Verification items for the finished model (mm, model axes). A direction names the side the tool comes from. Round coordinates to 2 decimals unless told otherwise and drop trailing zeros. Write each loop counter-clockwise with the first axis right and the second up, starting at its lowest first coordinate (ties: lowest second). Pieces come first, ordered by that corner, then holes. Notation, with made-up numbers: (31.25, 19) -> (78.25, 19) arc R27 ccw to (78.25, 37) -> close; hole circle Ø6 at (53.5, 77). An arc over 180 degrees is marked (long way). Answer as a JSON object with one key per item and string values. Group by question number.
(1) Gauge pin test, flat ends, axial feed: pin 1 Ø6 at (x, y) = (-55, -115) entering from -Z; pin 2 Ø1.5 at (x, y) = (-30.5, -43) entering from +Z; pin 3 Ø4.5 at (x, y) = (55, 115) entering from -Z. Record the tip position at first contact, or that the pin passes through.
(2) Draft check along Z on faces 1 (the face through (75, -2, 15)), 2 (the face through (24, 33, 0)), 3 (the face through (40, 125, -7)). Enter one of: released by +Z, released by -Z, zero draft, split by the parting line, or undercut.
(3) Scan lines: L1, parallel to Y at x = 50, z = 5.25; L2, parallel to Y at x = -55, z = 23.85; L3, parallel to X at y = 118, z = -12.5. Record each from-to range of solid material in increasing order. Write a range as from..to.
(4) Sectioned sample at A-A on z = 5.5. Count the separate pieces of the cut face and the enclosed holes in it, and give its area (3 significant figures).
(5) Sectioned sample at B-B on y = 97. Record the cut outline in (x, z), and give its area (3 significant figures).
(6) Set-up check for faces 4 (the face through (-54.227, 80.964, 4.93)), 5 (the face through (-1, 125, 15)), 6 (the face through (-80, -2, 5)), 7 (the face through (-29.46, -40.06, 23.52)), 8 (the face through (0, 29, -15)): record each of +Z, -Z, +X, -X, +Y, -Y from which the full face is reachable in a straight line by a thin tool's end or side.
(7) Sectioned sample at C-C on x = 65. Record the cut outline in (y, z), and give its area (3 significant figures).
```python
from build123d import *

# Parameters (mm, degrees)
CROQUIS1_W              = 150
CROQUIS1_H              = 250
CROQUIS1_R              = 19.5
SALIENTE_EXTRUIR1_DEPTH = 10
CROQUIS3_W              = 160
CROQUIS3_H              = 260
CROQUIS3_W_2            = 150
CROQUIS3_H_2            = 250
SALIENTE_EXTRUIR2_DEPTH = 25
SALIENTE_EXTRUIR3_DEPTH = 15
CROQUIS6_W              = 160
CROQUIS6_H              = 260
CROQUIS6_W_2            = 150
CROQUIS6_H_2            = 250
SALIENTE_EXTRUIR4_DEPTH = 15
CROQUIS7_W              = 160
CROQUIS7_H              = 260
SALIENTE_EXTRUIR5_DEPTH = 5
CROQUIS8_R              = 2.5
CORTAR_EXTRUIR1_DEPTH   = 3
CROQUIS9_R              = 2.5
CORTAR_EXTRUIR2_DEPTH   = 3


with BuildPart() as part:
    # Croquis1 → Saliente-Extruir1 (new body)
    with BuildSketch(Plane.XY):
        Rectangle(CROQUIS1_W, CROQUIS1_H)
        with Locations((-50, 100)):
            Circle(CROQUIS1_R, mode=Mode.SUBTRACT)
        with Locations((-50, 40)):
            Circle(CROQUIS1_R, mode=Mode.SUBTRACT)
        with Locations((-50, -20)):
            Circle(CROQUIS1_R, mode=Mode.SUBTRACT)
        with Locations(Location((50, -20, 0), (0, 0, 180))):
            Circle(CROQUIS1_R, mode=Mode.SUBTRACT)
        with Locations(Location((50, 40, 0), (0, 0, 180))):
            Circle(CROQUIS1_R, mode=Mode.SUBTRACT)
        with Locations(Location((50, 100, 0), (0, 0, 180))):
            Circle(CROQUIS1_R, mode=Mode.SUBTRACT)
        with Locations((-30, -100)):
            Circle(CROQUIS1_R, mode=Mode.SUBTRACT)
        with Locations(Location((30, -100, 0), (0, 0, 180))):
            Circle(CROQUIS1_R, mode=Mode.SUBTRACT)
        with Locations((0, -40)):
            Circle(CROQUIS1_R, mode=Mode.SUBTRACT)
    extrude(amount=SALIENTE_EXTRUIR1_DEPTH)

    # Croquis3 → Saliente-Extruir2 (add)
    with BuildSketch(Plane.XY.offset(10)):
        Rectangle(CROQUIS3_W, CROQUIS3_H)
        Rectangle(CROQUIS3_W_2, CROQUIS3_H_2, mode=Mode.SUBTRACT)
    extrude(amount=-SALIENTE_EXTRUIR2_DEPTH)

    # Croquis4 → Saliente-Extruir3 (add)
    with BuildSketch(Plane(origin=(0, 0, 0), x_dir=(-1, 0, 0), z_dir=(0, 0, -1))):
        Polygon((-5, 125), (-5, 5), (-75, -115), (-75, -125), (-3.830215177, -2.994654589), (3.830215177, -2.994654589), (75, -125), (75, -115), (4.127714662, 6.495346294), (5, 125), align=None)
    extrude(amount=SALIENTE_EXTRUIR3_DEPTH)

    # Croquis6 → Saliente-Extruir4 (add)
    with BuildSketch(Plane.XY.offset(10)):
        Rectangle(CROQUIS6_W, CROQUIS6_H)
        Rectangle(CROQUIS6_W_2, CROQUIS6_H_2, mode=Mode.SUBTRACT)
    extrude(amount=SALIENTE_EXTRUIR4_DEPTH)

    # Croquis7 → Saliente-Extruir5 (add)
    with BuildSketch(Plane.XY.offset(25)):
        Rectangle(CROQUIS7_W, CROQUIS7_H)
    extrude(amount=-SALIENTE_EXTRUIR5_DEPTH)

    # Croquis8 → Cortar-Extruir1 (cut)
    with BuildSketch(Plane.XY.offset(25)):
        with Locations((-30, 42.5)):
            Circle(CROQUIS8_R)
        with Locations(Location((-30, -42.5, 0), (0, 0, 180))):
            Circle(CROQUIS8_R)
    extrude(amount=-CORTAR_EXTRUIR1_DEPTH, mode=Mode.SUBTRACT)

    # Croquis9 → Cortar-Extruir2 (cut)
    with BuildSketch(Plane.XY.offset(25)):
        with Locations((-55, 115)):
            Circle(CROQUIS9_R)
        with Locations(Location((55, 115, 0), (0, 0, 180))):
            Circle(CROQUIS9_R)
        with Locations((55, -115)):
            Circle(CROQUIS9_R)
        with Locations(Location((-55, -115, 0), (0, 0, 180))):
            Circle(CROQUIS9_R)
    extrude(amount=-CORTAR_EXTRUIR2_DEPTH, mode=Mode.SUBTRACT)


solid = part.part
```
Computed values:
{
 "1": {"pin 1": "z = 0", "pin 2": "z = 22", "pin 3": "z = 20"},
 "2": {"face 1": "undercut", "face 2": "released by -Z", "face 3": "zero draft"},
 "3": {"L1": "-130..-39.5, -0.5..20.5, 59.5..80.5, 119.5..130", "L2": "-130..-117.5, -112.5..112.5, 117.5..130", "L3": "-80..-75, -4.95..5, 75..80"},
 "4": {"separate pieces": "1", "enclosed holes": "9", "area": "30,800 mm2"},
 "5": {"outline": "(-80, -15) -> (-75, -15) -> (-75, 0) -> (-69.27, 0) -> (-69.27, 10) -> (-75, 10) -> (-75, 20) -> (75, 20) -> (75, 10) -> (69.27, 10) -> (69.27, 0) -> (75, 0) -> (75, -15) -> (80, -15) -> (80, 25) -> (-80, 25) -> close; (-30.73, 0) -> (-4.79, 0) -> (-4.79, -15) -> (5, -15) -> (5, 0) -> (30.73, 0) -> (30.73, 10) -> (-30.73, 10) -> close", "area": "2,030 mm2"},
 "6": {"face 4": "-Z", "face 5": "none", "face 6": "+Z, -Z, -X, +Y, -Y", "face 7": "+Z", "face 8": "-Z, +X, -X, +Y, -Y"},
 "7": {"outline": "(-130, -15) -> (-125, -15) -> (-125, 0) -> (-107.86, 0) -> (-107.86, -15) -> (-97.86, -15) -> (-97.86, 0) -> (-32.46, 0) -> (-32.46, 10) -> (-125, 10) -> (-125, 20) -> (125, 20) -> (125, 10) -> (112.46, 10) -> (112.46, 0) -> (125, 0) -> (125, -15) -> (130, -15) -> (130, 25) -> (-130, 25) -> close; (-7.54, 0) -> (27.54, 0) -> (27.54, 10) -> (-7.54, 10) -> close; (52.46, 0) -> (87.54, 0) -> (87.54, 10) -> (52.46, 10) -> close", "area": "3,550 mm2"}
}
